```python
from build123d import *

# Parameters (mm, degrees)
BOSS_EXTRU_1_DEPTH      = 95
ESQUISSE2_W             = 15
ESQUISSE2_H             = 5.425563258
ENL_V_MAT_EXTRU_1_DEPTH = 46


with BuildPart() as part:
    # Esquisse1 → Boss.-Extru.1 (new body)
    with BuildSketch(Plane.XY):
        Polygon((-27.258684463, 5.425563258), (-27.258684463, 0), (2.741315537, 0), (2.741315537, 5.425563258), (0.741315537, 5.425563258), (0.741315537, 2), (-25.258684463, 2), (-25.258684463, 5.425563258), align=None)
    extrude(amount=BOSS_EXTRU_1_DEPTH)

    # Esquisse2 → Enlèv. mat.-Extru.1 (cut)
    with BuildSketch(Plane(origin=(2.741315537, 0, 0), x_dir=(0, 0, -1), z_dir=(1, 0, 0))):
        with Locations((-87.5, 2.712781629)):
            Rectangle(ESQUISSE2_W, ESQUISSE2_H)
    extrude(amount=-ENL_V_MAT_EXTRU_1_DEPTH, mode=Mode.SUBTRACT)


solid = part.part
```
Part model, mm, in its own coordinate system. A direction names the side the tool comes from. Give positions to 0.01 mm unless a question says otherwise; leave off trailing zeros. Write each loop counter-clockwise with the first axis right and the second up, starting at its lowest first coordinate (ties: lowest second). Pieces come first, ordered by that corner, then holes. Notation, with made-up numbers: (33, 16) -> (92, 16) arc R18 cw to (92, 37) -> close; hole circle Ø3 at (26, 3). An arc over 180 degrees is marked (long way). Put each result on its own line as item: value. Start each with the question number.
Item 1: Cut at A-A (y = 2.8). List the corners of the cut face in (x, z).
Item 2: Pull direction X, two halves, no side cores. Call faces 1 (the face through (-25.259, 4, 39)), 2 (the face through (0.741, 4, 39)), 3 (the face through (-12, 1, 80)), 4 (the face through (-27.259, 3, 39)): pulls with the +X half, pulls with the -X half, needs draft (parallel to the pull), parting line crosses it, or undercut.
Item 3: Which spindle directions (+Z, -Z, +X, -X, +Y, -Y) get a long thin tool onto all of the face, cutting with end or side? Do faces 5 (the face through (-12, 2, 39)), 6 (the face through (2.741, 3, 39)). Say none if no direction does.
Item 4: Cut at C-C (x = -2.25). List the corners of the cut face in (y, z), then the cut area to 3 significant figures.
Item 5: Pin check, flat tips, straight feed: pin 1 Ø8 at (x, z) = (-10.5, 21) entering from +Y; pin 2 Ø2 at (x, y) = (-15.5, 1) entering from -Z. Stop position of each tip, or through.
Item 6: Wall check: L1, parallel to X at y = 5.1, z = 48.5; L2, parallel to Y at x = -22.25, z = 7.5. Give the ranges that are in metal, low to high. Write a range as [from, to].
Item 7: Cut at B-B (z = 58). List the corners of the cut face in (x, y), then the cut area to 3 significant figures.
Answer list:
1. outline: (-27.26, 0) -> (-25.26, 0) -> (-25.26, 80) -> (-27.26, 80) -> close; (0.74, 0) -> (2.74, 0) -> (2.74, 80) -> (0.74, 80) -> close
2. face 1: undercut
2. face 2: undercut
2. face 3: needs draft
2. face 4: pulls with the -X half
3. face 5: +Z, -Z, +Y
3. face 6: +Z, -Z, +X, +Y, -Y
4. outline: (0, 0) -> (2, 0) -> (2, 80) -> (0, 80) -> close
4. area: 160 mm2
5. pin 1: stops at y = 2
5. pin 2: stops at z = 0
6. L1: x = [-27.26, -25.26], [0.74, 2.74]
6. L2: y = [0, 2]
7. outline: (-27.26, 0) -> (2.74, 0) -> (2.74, 5.43) -> (0.74, 5.43) -> (0.74, 2) -> (-25.26, 2) -> (-25.26, 5.43) -> (-27.26, 5.43) -> close
7. area: 73.7 mm2
